Answer from the drawing. Dimensions are ordinates in mm from the lowest x, y and z of the part. Give positions to 0.01 mm unless a question says otherwise; leave off trailing zeros. Write each loop counter-clockwise with the first axis right and the second up, starting at its lowest first coordinate (ties: lowest second). Pieces come first, ordered by that corner, then holes. Notation, with made-up numbers: M 71,64 L 116,64 A19 ccw 116,101 Z; hole C 74,23 d3. An arc over 180 degrees is marked long. Put each result on its own line as item: value.
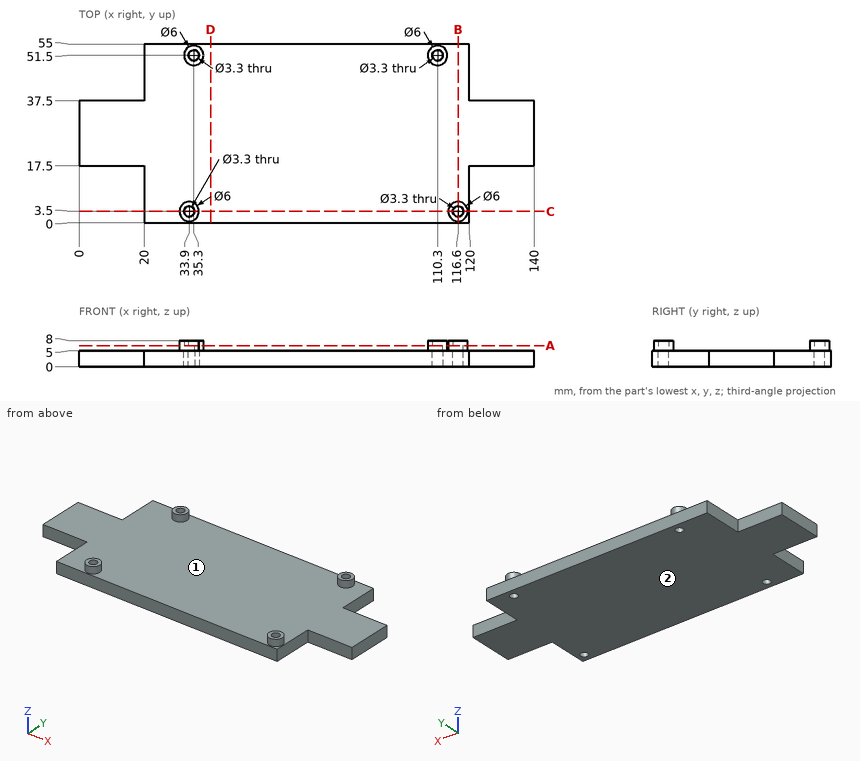
(1) Straight lines are drawn through the part: line 1 along Y through (x, z) = (116.6, 3); line 2 along Y through (x, z) = (33.9, 6.1); line 3 along X through (y, z) = (3, 3). For each, find the intervals that lie inside material, in ascending order. Write a range as from..to.
Result:
line 1: y = 0..1.85, 5.15..55
line 2: y = 0.5..1.85, 5.15..6.5, 48.85..50.63, 52.37..54.15
line 3: x = 20..32.33, 35.47..115.03, 118.17..120
(2) Given pin 1 Ø1.5 at (x, z) = (13.5, 3.5) entering from -Y; pin 2 Ø3 at (x, y) = (33.9, 3.5) entering from +Z; pin 3 Ø2.5 at (y, z) = (6.5, 3) entering from -X; pin 4 Ø4.5 at (x, y) = (116.6, 3.5) entering from +Z, each flat-ended and moving along its own axis, determine where each tip first touches the part or whether it passes through.
Result:
pin 1: stops at y = 17.5
pin 2: passes through
pin 3: stops at x = 20
pin 4: stops at z = 8
(3) Section B-B on x = 116.6 is taken. Determine the outline of the cut face in (y, z).
Result:
outline: M 0,0 L 1.85,0 L 1.85,8 L 0.5,8 L 0.5,5 L 0,5 Z; M 5.15,0 L 55,0 L 55,5 L 6.5,5 L 6.5,8 L 5.15,8 Z
(4) For a pull along X with two mould halves and no side action, classify the marked faces 1 and 2 as +X half, -X half, draft (parallel to the pull), parting line (faces both ways), or undercut.
Result:
face 1: undercut
face 2: draft
(5) Section D-D on x = 40.5 is taken. Determine the outline of the cut face in (y, z), and give its area (3 significant figures).
Result:
outline: M 0,0 L 55,0 L 55,5 L 0,5 Z
area: 275 mm²
(6) Section C-C on y = 3.5 is taken. Determine the outline of the cut face in (x, z), and give its area (3 significant figures).
Result:
outline: M 20,0 L 32.25,0 L 32.25,8 L 30.9,8 L 30.9,5 L 20,5 Z; M 35.55,0 L 114.95,0 L 114.95,8 L 113.6,8 L 113.6,5 L 36.9,5 L 36.9,8 L 35.55,8 Z; M 118.25,0 L 120,0 L 120,5 L 119.6,5 L 119.6,8 L 118.25,8 Z
area: 483 mm²
(7) Section A-A on z = 6.5 is taken. Determine the outline of the cut face in (x, y).
Result:
outline: C 33.9,3.5 d6; C 35.3,51.5 d6; C 110.3,51.5 d6; C 116.6,3.5 d6; hole C 33.9,3.5 d3.3; hole C 35.3,51.5 d3.3; hole C 110.3,51.5 d3.3; hole C 116.6,3.5 d3.3
